Can you work these out from the model? Positions are in its coordinate system, mm. A direction names the side the tool comes from. Coordinates: 2 decimals unless noted, no trailing zeros. Write each loop counter-clockwise with the first axis right and the second up, starting at its lowest first coordinate (ties: lowest second). Pieces come first, ordered by that corner, then holes. Notation, with made-up numbers: M 9.25,55 L 63.25,55 A21 cw 63.25,76 Z; hole C 71,44.25 d5. An arc over 180 degrees is marked long. Answer as a JSON object with one key per item and string values. Group by question number.
from build123d import *

# Parameters (mm, degrees)
SKETCH_1_W          = 200
SKETCH_1_H          = 270
EXTRUDE_1_DEPTH     = 10
SKETCH_3_R          = 2.5
CUT_EXTRUDE_1_DEPTH = 20
SKETCH_6_W          = 90
SKETCH_6_H          = 50
EXTRUDE_2_DEPTH     = 30
CUT_EXTRUDE_3_REACH = 339.343
SKETCH_9_W          = 17
SKETCH_9_H          = 25
EXTRUDE_4_DEPTH     = 15
SKETCH_11_R         = 2
CUT_EXTRUDE_4_DEPTH = 8
SKETCH_12_R         = 2.5
EXTRUDE_5_DEPTH     = 25


with BuildPart() as part:
    # 草图1 → 凸台-拉伸1 (new body)
    with BuildSketch(Plane(origin=(0, 0, 0), x_dir=(1, 0, 0), z_dir=(0, 1, 0))):
        with Locations((100, 135)):
            Rectangle(SKETCH_1_W, SKETCH_1_H)
    extrude(amount=EXTRUDE_1_DEPTH)

    # 草图3 → 切除-拉伸1 (cut)
    with BuildSketch(Plane(origin=(0, 10, 0), x_dir=(1, 0, 0), z_dir=(0, 1, 0))):
        with Locations(Location((10, 260, 0), (0, 0, 270))):
            Circle(SKETCH_3_R)
        with Locations(Location((10, 10, 0), (0, 0, 270))):
            Circle(SKETCH_3_R)
        with Locations(Location((190, 10, 0), (0, 0, 270))):
            Circle(SKETCH_3_R)
        with Locations(Location((190, 260, 0), (0, 0, 270))):
            Circle(SKETCH_3_R)
    extrude(amount=-CUT_EXTRUDE_1_DEPTH, mode=Mode.SUBTRACT)

    # 草图6 → 凸台-拉伸2 (add)
    with BuildSketch(Plane(origin=(0, 10, 0), x_dir=(1, 0, 0), z_dir=(0, 1, 0))):
        with Locations((105, 135)):
            Rectangle(SKETCH_6_W, SKETCH_6_H)
    extrude(amount=EXTRUDE_2_DEPTH)

    # 草图9 → 切除-拉伸3 (cut, up to next)
    with BuildSketch(Plane(origin=(0, 10, 0), x_dir=(1, 0, 0), z_dir=(0, 1, 0)), mode=Mode.PRIVATE) as cut_extrude_3_sk1:
        with Locations((66.5, 172.5)):
            Rectangle(SKETCH_9_W, SKETCH_9_H)
    cut_extrude_3_tool1 = extrude(cut_extrude_3_sk1.sketch, amount=-CUT_EXTRUDE_3_REACH, mode=Mode.PRIVATE) & part.part
    add(cut_extrude_3_tool1.solids().sort_by_distance((66.5, 10, -172.5))[0], mode=Mode.SUBTRACT)

    # 草图5 → 凸台-拉伸4 (add, symmetric)
    with BuildSketch(Plane(origin=(100, 0, 0), x_dir=(0, 0, -1), z_dir=(1, 0, 0))):
        Polygon((232.5, 10), (232.5, 11), (242.5, 11), (242.5, 10), (252.5, 10), (252.5, 11), (243.5, 11), (243.5, 12), (231.5, 12), (231.5, 11), (222.5, 11), (222.5, 10), align=None)
    extrude(amount=EXTRUDE_4_DEPTH, both=True)

    # 草图11 → 切除-拉伸4 (cut)
    with BuildSketch(Plane(origin=(0, 11, 0), x_dir=(1, 0, 0), z_dir=(0, 1, 0))):
        with Locations(Location((90, 227.5, 0), (0, 0, 270))):
            Circle(SKETCH_11_R)
        with Locations(Location((110, 227.5, 0), (0, 0, 270))):
            Circle(SKETCH_11_R)
        with Locations(Location((90, 247.5, 0), (0, 0, 270))):
            Circle(SKETCH_11_R)
        with Locations(Location((110, 247.5, 0), (0, 0, 270))):
            Circle(SKETCH_11_R)
    extrude(amount=-CUT_EXTRUDE_4_DEPTH, mode=Mode.SUBTRACT)

    # 草图12 → 凸台-拉伸5 (add)
    with BuildSketch(Plane(origin=(0, 0, -160), x_dir=(-1, 0, 0), z_dir=(0, 0, -1))):
        with Locations(Location((-78, 25, 0), (0, 0, 180))):
            Circle(SKETCH_12_R)
    extrude(amount=EXTRUDE_5_DEPTH)


solid = part.part
Q1. Please list where these lines run through material, in increasing order: L1, parallel to Z at x = 190, y = 7.75; L2, parallel to X at y = 7.5, z = -247.5; L3, parallel to X at y = 8, z = -10.
Q2. If we section it at C-C on z = -141: List the corners of the cut face in (x, y) for me, and give its area (3 significant figures).
Q3. We'd pull the mould along Z, two halves only. Please class faces 6 (the flat face through (0, 5, -133)), 7 (the flat face through (100, 11, -237)), 8 (the flat face through (104, 25, -110)), 9 (the flat face through (99, 5, -270)): pulls with the +Z half, pulls with the -Z half, needs draft (parallel to the pull), parting line crosses it, or undercut.
Q4. If we section it at B-B on x = 102: List the corners of the cut face in (y, z) for me.
Q5. Will these pins go through, and if not, where does the flat tip stop? pin 1 (2 mm diameter, centred on y = 14, z = -130.5, fed in from -X); pin 2 (10 mm diameter, centred on x = 97.5, z = -227, fed in from +Y); pin 3 (1 mm diameter, centred on x = 60, z = -51.5, fed in from +Y).
Q6. If we section it at A-A on x = 69: List the corners of the cut face in (y, z) for me, and give its area (3 significant figures).
Q7. If we section it at D-D on y = 18.5: List the corners of the cut face in (x, z) for me, and give its area (3 significant figures).
Q8. On a 3-axis mill with a long thin cutter (end or side, diameter ignored), from which of +Z, -Z, +X, -X, +Y, -Y can I reach the whole of each face in a straight line? I mean faces 1 (the flat face through (75, 5, -172)), 2 (the flat face through (150, 25, -135)), 3 (the flat face through (100, 11, -227)), 4 (the flat face through (100, 11, -248)), 5 (the flat face through (60, 25, -135)). Say none if no direction works.
Reply:
{
 "1": {"L1": "-270 to -262.5, -257.5 to -12.5, -7.5 to 0", "L2": "0 to 88, 92 to 108, 112 to 200", "L3": "0 to 7.5, 12.5 to 187.5, 192.5 to 200"},
 "2": {"outline": "M 0,0 L 200,0 L 200,10 L 150,10 L 150,40 L 60,40 L 60,10 L 0,10 Z", "area": "4,700 mm^2"},
 "3": {"face 6": "needs draft", "face 7": "undercut", "face 8": "pulls with the +Z half", "face 9": "pulls with the -Z half"},
 "4": {"outline": "M 0,-270 L 10,-270 L 10,-252.5 L 11,-252.5 L 11,-243.5 L 12,-243.5 L 12,-231.5 L 11,-231.5 L 11,-222.5 L 10,-222.5 L 10,-160 L 40,-160 L 40,-110 L 10,-110 L 10,0 L 0,0 Z; hole M 10,-242.5 L 11,-242.5 L 11,-232.5 L 10,-232.5 Z"},
 "5": {"pin 1": "x = 60", "pin 2": "y = 12", "pin 3": "y = 10"},
 "6": {"outline": "M 0,-270 L 10,-270 L 10,-185 L 0,-185 Z; M 0,-160 L 40,-160 L 40,-110 L 10,-110 L 10,0 L 0,0 Z", "area": "3,950 mm^2"},
 "7": {"outline": "M 60,-160 L 150,-160 L 150,-110 L 60,-110 Z", "area": "4,500 mm^2"},
 "8": {"face 1": "+Y, -Y", "face 2": "+Z, -Z, +X, +Y", "face 3": "+X, -X, +Y", "face 4": "-Z, +X, -X, +Y", "face 5": "+Z, -Z, -X, +Y"}
}
